```python
from build123d import *


with BuildPart() as part:
    # Sketch1 → Revolve1 (revolve)
    with BuildSketch(Plane.XY):
        with BuildLine():
            Line((0, 0), (0, 12.5))
            ThreePointArc((0, 12.5), (0.146446609, 12.853553391), (0.5, 13))
            Line((0.5, 13), (89.5, 13))
            ThreePointArc((89.5, 13), (89.853553391, 12.853553391), (90, 12.5))
            Line((90, 12.5), (90, 11.2))
            ThreePointArc((90, 11.2), (90.058578644, 11.058578644), (90.2, 11))
            Line((90.2, 11), (103, 11))
            Line((103, 11), (103, 10.5))
            Line((103, 10.5), (104.3, 10.5))
            Line((104.3, 10.5), (104.3, 11))
            Line((104.3, 11), (107, 11))
            ThreePointArc((107, 11), (107.353553391, 10.853553391), (107.5, 10.5))
            Line((107.5, 10.5), (107.5, 0))
            Line((107.5, 0), (0, 0))
        make_face()
    revolve(axis=Axis((0, 0, 0), (1, 0, 0)))


solid = part.part
```
Geometry check sheet. Reference: the model listing, model coordinates, mm. A direction names the side the tool comes from. Round coordinates to 2 decimals unless told otherwise and drop trailing zeros. Loops run counter-clockwise (first coordinate to the right, second up) from the corner with the lowest first, then second, coordinate; pieces in that order, holes last. Notation, with made-up numbers: (77, -39.75) - (132, -39.75) arc R25 cw to (132, -23.75) - close; hole circle Ø5 at (47.5, -24.75). An arc over 180 degrees is marked (long way). Write each question's results on one line, items separated by ' | '. Start each with the question number.
Q1. Thickness scan on line 1 (X direction, y = 10.5, z = -1); line 2 (Y direction, x = 87, z = -0.5); line 3 (Y direction, x = 26, z = -3.5). Record the ranges inside material, lowest first. Write a range as [from, to].
Q2. Access from +Z, -Z, +X, -X, +Y, -Y to the whole of each face (thin tool, end or side, straight path). Record for faces 4 (the cylindrical face through (96.69, -2.38, -10.74)), 5 (the flat face through (107.5, 0, 0)), 6 (the flat face through (103, 10, -4)).
Q3. Gauge pin test, flat ends, axial feed: P1, Ø3, axis at y = -9.5, z = -9, coming from the +X side; P2, Ø5, axis at x = 16.5, y = -8.5, coming from the +Z side; P3, Ø3, axis at x = 19, z = 7, coming from the +Y side; P4, Ø12, axis at x = 80.5, y = 1.5, coming from the +Z side. Record the tip position at first contact, or that the pin passes through.
Q4. Cross-section at C-C on x = 19.5. Enter the section's corners in (y, z).
Q5. Release check for a two-part mould opening along X. For faces 1 (the cylindrical face through (103.7, 10, 3.2)), 2 (the cylindrical face through (105.67, -2.38, -10.74)), 3 (the flat face through (90, -11.2, 1.9)) record: +X half, -X half, draft (parallel to the pull), parting line (faces both ways), or undercut.
Q6. Cross-section at D-D on x = 93.5. Enter the section's corners in (y, z).
Q7. Cross-section at A-A on z = 0. Enter the section's corners in (x, y).
Answers below:
1) line 1: x = [0, 103], [104.3, 107.5] | line 2: y = [-12.99, 12.99] | line 3: y = [-12.52, 12.52]
2) face 4: +X | face 5: +Z, -Z, +X, +Y, -Y | face 6: none
3) P1: stops at x = 90 | P2: stops at z = 11.53 | P3: stops at y = 11.78 | P4: stops at z = 13
4) outline: circle Ø26 at (0, 0)
5) face 1: undercut | face 2: draft | face 3: +X half
6) outline: circle Ø22 at (0, 0)
7) outline: (0, -12.5) arc R0.5 ccw to (0.5, -13) - (89.5, -13) arc R0.5 ccw to (90, -12.5) - (90, -11.2) arc R0.2 cw to (90.2, -11) - (103, -11) - (103, -10.5) - (104.3, -10.5) - (104.3, -11) - (107, -11) arc R0.5 ccw to (107.5, -10.5) - (107.5, 10.5) arc R0.5 ccw to (107, 11) - (104.3, 11) - (104.3, 10.5) - (103, 10.5) - (103, 11) - (90.2, 11) arc R0.2 cw to (90, 11.2) - (90, 12.5) arc R0.5 ccw to (89.5, 13) - (0.5, 13) arc R0.5 ccw to (0, 12.5) - close
